from build123d import *

# Parameters (mm, degrees)
F1_DEPTH = 11
F0_R     = 1
F2_DEPTH = 1


with BuildPart() as f1:
    # F0 (on Top) → F1 (new body)
    with BuildSketch(Plane.XY):
        Polygon((-2.984679, 1.723205), (-2.984679, -1.723205), (0, -3.44641), (2.984679, -1.723205), (2.984679, 1.723205), (0, 3.44641), align=None)
        Polygon((0, 3.1), (2.684679, 1.55), (2.684679, -1.55), (0, -3.1), (-2.684679, -1.55), (-2.684679, 1.55), align=None, mode=Mode.SUBTRACT)
    extrude(amount=F1_DEPTH)

    # F0 (on Top) → F2 (join)
    with BuildSketch(Plane.XY):
        Polygon((2.684679, -1.55), (2.684679, 1.55), (0, 3.1), (-2.684679, 1.55), (-2.684679, -1.55), (0, -3.1), align=None)
        Circle(F0_R, mode=Mode.SUBTRACT)
    extrude(amount=F2_DEPTH)


solid = f1.part
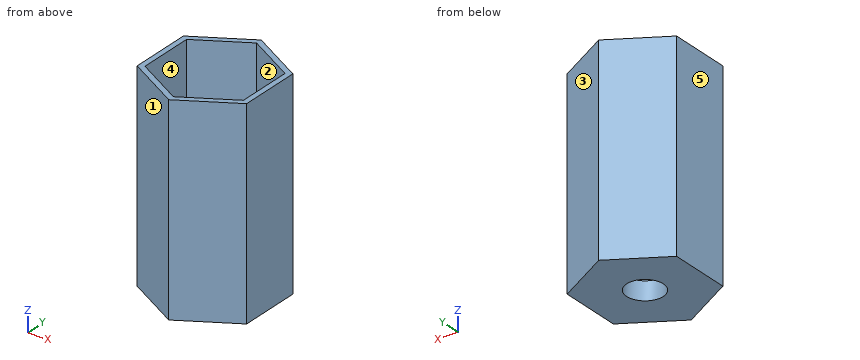
Geometry: final body of the model. Coordinates: model frame, mm. Face numbers are marked on the shaded views. A direction names the side the tool comes from. Round coordinates to 2 decimals unless told otherwise and drop trailing zeros. Loops run counter-clockwise (first coordinate to the right, second up) from the corner with the lowest first, then second, coordinate; pieces in that order, holes last.
Q1. Section C-C on y = 1.25. Return loops of the section in (x, z).
Q2. Section B-B on z = 3. Return loops of the section in (x, y), plus the area to 3 significant figures.
Q3. Section A-A on y = 0. Return loops of the section in (x, z).
Q4. Pin query (flat end, axial travel): P1, Ø1, axis at x = -2, z = 3, coming from the -Y side; P2, Ø2.5, axis at x = 0, y = 0, coming from the +Z side; P3, Ø1.5, axis at y = -2, z = 9.5, coming from the +X side; P4, Ø1.5, axis at x = 1, z = 5, coming from the -Y side. Return the tip coordinate at first contact, or that it passes through.
Q5. Access query for the marked faces 1 and 2. Directions: +Z, -Z, +X, -X, +Y, -Y. A direction counts if a zero-diameter tool reaches every point of the face in a straight line with its end or side. Return the directions, or none.
Q6. Section D-D on x = -0.7. Return loops of the section in (y, z).
Q7. Material intervals for L1, parallel to Y at x = -2.1, z = 7.5; L2, parallel to X at y = -0.5, z = 10.5; L3, parallel to Y at x = 1.9, z = 7.75, sorted ascending.
Q8. Pull-direction query (X, two-part tool) for the marked faces 3, 4 and 5; classes: released by +X, released by -X, zero draft, split by the parting line, or undercut.
Evaluation:
1. outline: (-2.98, 0) - (2.98, 0) - (2.98, 11) - (2.68, 11) - (2.68, 1) - (-2.68, 1) - (-2.68, 11) - (-2.98, 11) - close
2. outline: (-2.98, -1.72) - (0, -3.45) - (2.98, -1.72) - (2.98, 1.72) - (0, 3.45) - (-2.98, 1.72) - close; hole (-2.68, -1.55) - (0, -3.1) - (2.68, -1.55) - (2.68, 1.55) - (0, 3.1) - (-2.68, 1.55) - close
2. area: 5.89 mm2
3. outline: (-2.98, 0) - (-1, 0) - (-1, 1) - (-2.68, 1) - (-2.68, 11) - (-2.98, 11) - close; (1, 0) - (2.98, 0) - (2.98, 11) - (2.68, 11) - (2.68, 1) - (1, 1) - close
4. P1: stops at y = -2.58
4. P2: stops at z = 1
4. P3: stops at x = 2.98
4. P4: stops at y = -3.3
5. face 1: +Z, -Z, -X, -Y
5. face 2: +Z
6. outline: (-3.04, 0) - (-0.71, 0) - (-0.71, 1) - (-2.7, 1) - (-2.7, 11) - (-3.04, 11) - close; (0.71, 0) - (3.04, 0) - (3.04, 11) - (2.7, 11) - (2.7, 1) - (0.71, 1) - close
7. L1: y = -2.23 to -1.89, 1.89 to 2.23
7. L2: x = -2.98 to -2.68, 2.68 to 2.98
7. L3: y = -2.35 to -2, 2 to 2.35
8. face 3: released by +X
8. face 4: undercut
8. face 5: released by -X
